CAD build for the part. Positions are in the model's coordinates, mm. A direction names the side the tool comes from. Round coordinates to 2 decimals unless told otherwise and drop trailing zeros. Order: outer loops, then holes, each group sorted by start corner. A loop starts at its lowest first (then second) coordinate and runs counter-clockwise, first axis right, second up. Notation, with made-up numbers: (-31.5, 24.5) -> (13.5, 24.5) arc R11 ccw to (13.5, 44.5) -> close; hole circle Ø11 at (-32.5, 52). An arc over 180 degrees is marked (long way). Answer as CSV lines item,"result". Start each with the question number.
from build123d import *

# Parameters (mm, degrees)
EXTRUSION1_DEPTH      = 43
EXTRUSION1_DEPTH_BACK = 43
EXTRUSION2_DEPTH      = 49


with BuildPart() as part:
    # Esquisse1 → Extrusion1 (new, two sides: drawn at the far end of the back side and taken through both)
    with BuildSketch(Plane(origin=(0, 0, 0), x_dir=(1, 0, 0), z_dir=(0, 1, 0)).offset(-EXTRUSION1_DEPTH_BACK)):
        with BuildLine():
            Line((43, 0), (-90, 0))
            Line((-90, 0), (-289.512810052, 13.951294749))
            ThreePointArc((-289.512810052, 13.951294749), (-292.060894193, 13.374722173), (-293.867473702, 11.487544597))
            Line((-293.867473702, 11.487544597), (-295.268797801, 8.737291199))
            ThreePointArc((-295.268797801, 8.737291199), (-296.837030139, 7.099094327), (-299.048938294, 6.59859061))
            Line((-299.048938294, 6.59859061), (-368.878421812, 11.481543773))
            Line((-368.878421812, 11.481543773), (-368.878421812, 14.488869467))
            Line((-368.878421812, 14.488869467), (-298.839668873, 9.591282761))
            ThreePointArc((-298.839668873, 9.591282761), (-298.314300819, 9.710161415), (-297.941817373, 10.099262699))
            Line((-297.941817373, 10.099262699), (-296.540493275, 12.849516097))
            ThreePointArc((-296.540493275, 12.849516097), (-293.538164873, 15.985789261), (-289.303540631, 16.9439869))
            Line((-289.303540631, 16.9439869), (-283.5, 16.538163805))
            Line((-283.5, 16.538163805), (-283.5, 52))
            Line((-283.5, 52), (-261.5, 52))
            Line((-261.5, 52), (-261.5, 14.999773943))
            Line((-261.5, 14.999773943), (-89.895237692, 3))
            Line((-89.895237692, 3), (43, 3))
            Line((43, 3), (43, 0))
        make_face()
    extrude(amount=EXTRUSION1_DEPTH + EXTRUSION1_DEPTH_BACK)

    # Esquisse2 → Extrusion2 (add)
    with BuildSketch(Plane(origin=(0, 0, -3), x_dir=(-1, 0, 0), z_dir=(0, 0, -1))):
        with BuildLine():
            Line((27, 43), (27, 40))
            Line((27, 40), (36, 40))
            ThreePointArc((36, 40), (39.473291852, 38.596699002), (40.996954135, 35.174497484))
            Line((40.996954135, 35.174497484), (41.666542342, 16))
            ThreePointArc((41.666542342, 16), (42.545221998, 13.878679656), (44.666542342, 13))
            Line((44.666542342, 13), (56.368378428, 13))
            ThreePointArc((56.368378428, 13), (58.459244141, 13.909134287), (59.368378428, 16))
            Line((59.368378428, 16), (60.003045865, 34.174497484))
            ThreePointArc((60.003045865, 34.174497484), (61.526708148, 37.596699002), (65, 39))
            Line((65, 39), (65, 43))
            Line((65, 43), (27, 43))
        make_face()
    extrude(amount=EXTRUSION2_DEPTH)


solid = part.part
Item 1: Pin check, flat tips, straight feed: pin 1 (10 mm diameter, centred on x = -32, z = -25.5, fed in from -Y); pin 2 (4.5 mm diameter, centred on y = 41, z = -34.5, fed in from -X); pin 3 (2 mm diameter, centred on x = -63.5, y = -32, fed in from -Z). Stop position of each tip, or through.
Item 2: Band-saw the part on B-B, the plane y = -4. Give the cut face in (x, z), and give its area (3 significant figures).
Item 3: Mould opens along X. For faces 1 (the flat face through (-333.475, -0.602, -9.006)), 2 (the flat face through (-188.36, -0.6, -6.88)), 3 (the flat face through (-208, -43, -11)) say: released by +X, released by -X, zero draft, split by the parting line, or undercut.
Item 4: Tool access for faces 4 (the flat face through (-273, -1, -52)), 5 (the flat face through (-50, 13, -27)), 6 (the flat face through (-334.349, -0.602, -12.074)): list every direction of +Z, -Z, +X, -X, +Y, -Y with a clear straight run to the whole face (end or side of a thin tool).
Item 5: Probe line 1 (X direction, y = -31, z = -28.5); line 2 (X direction, y = 16.5, z = -45.5); line 3 (X direction, y = 37.5, z = -35). List the from-to ranges inside material, lowest first.
Item 6: Band-saw the part on D-D, the plane y = 29.5. Give the cut face in (x, z).
Item 7: Band-saw the part on C-C, the plane x = -75.5. Give the cut face in (y, z), and give its area (3 significant figures).
Item 8: Band-saw the part on A-A, the plane z = -22. Give the cut face in (x, y), and give its area (3 significant figures).
Values:
1,pin 1,"y = 39.9"
1,pin 2,"x = -283.5"
1,pin 3,"z = -3"
2,outline,"(-368.88, -14.49) -> (-298.84, -9.59) arc R0.93 cw to (-297.94, -10.1) -> (-296.54, -12.85) arc R7.53 ccw to (-289.3, -16.94) -> (-283.5, -16.54) -> (-283.5, -52) -> (-261.5, -52) -> (-261.5, -15) -> (-89.9, -3) -> (43, -3) -> (43, 0) -> (-90, 0) -> (-289.51, -13.95) arc R4.53 cw to (-293.87, -11.49) -> (-295.27, -8.74) arc R3.93 ccw to (-299.05, -6.6) -> (-368.88, -11.48) -> close"
2,area,"2,050 mm²"
3,face 1,"released by -X"
3,face 2,"undercut"
3,face 3,"zero draft"
4,face 4,"-Z, +X, -X, +Y, -Y"
4,face 5,"-Z, +X, -Y"
4,face 6,"-Z, +Y, -Y"
5,line 1,"-283.5 to -261.5"
5,line 2,"-283.5 to -261.5, -59.39 to -41.65"
5,line 3,"-283.5 to -261.5, -61.43 to -40.33"
6,outline,"(-368.88, -14.49) -> (-298.84, -9.59) arc R0.93 cw to (-297.94, -10.1) -> (-296.54, -12.85) arc R7.53 ccw to (-289.3, -16.94) -> (-283.5, -16.54) -> (-283.5, -52) -> (-261.5, -52) -> (-261.5, -15) -> (-89.9, -3) -> (-59.84, -3) -> (-59.84, -52) -> (-41.2, -52) -> (-41.2, -3) -> (43, -3) -> (43, 0) -> (-90, 0) -> (-289.51, -13.95) arc R4.53 cw to (-293.87, -11.49) -> (-295.27, -8.74) arc R3.93 ccw to (-299.05, -6.6) -> (-368.88, -11.48) -> close"
7,outline,"(-43, -3) -> (43, -3) -> (43, 0) -> (-43, 0) -> close"
7,area,"258 mm²"
8,outline,"(-283.5, -43) -> (-261.5, -43) -> (-261.5, 43) -> (-283.5, 43) -> close; (-65, 39) arc R5 cw to (-60, 34.17) -> (-59.37, 16) arc R3.11 ccw to (-56.37, 13) -> (-44.67, 13) arc R3 ccw to (-41.67, 16) -> (-41, 35.17) arc R5 cw to (-36, 40) -> (-27, 40) -> (-27, 43) -> (-65, 43) -> close"
8,area,"2,510 mm²"
